Build history of the part. All positions in model axes, mm. Give positions to 0.01 mm unless a question says otherwise; leave off trailing zeros. Order: outer loops, then holes, each group sorted by start corner. A loop starts at its lowest first (then second) coordinate and runs counter-clockwise, first axis right, second up. Notation, with made-up numbers: M -5,28 L 44,28 A12 ccw 44,46 Z; hole C -38.5,84.25 d2. An arc over 180 degrees is marked long. Use CSV: the item, a comma, the result in double quotes. Start each with the question number.
Item 1: Wall check: line 1 along Y through (x, z) = (-2, -2.75); line 2 along X through (y, z) = (3.4, 2.5); line 3 along Z through (x, y) = (6.25, 0.2). Give the ranges that are in metal, low to high.
Item 2: Band-saw the part on A-A on z = 3. Write the cut outline in (x, y), plus the area to 3 significant figures.
Item 3: Pin check, flat tips, straight feed: P1, Ø2, axis at y = 3.5, z = 4, coming from the -X side; P2, Ø1, axis at x = 3.5, y = 1.5, coming from the -Z side; P3, Ø1.5, axis at x = 1.5, z = 4, coming from the -Y side; P4, Ø1.5, axis at y = 1, z = -4, coming from the -X side. Stop position of each tip, or through.
Item 4: Band-saw the part on D-D on y = 1.35. Write the cut outline in (x, z), plus the area to 3 significant figures.
Item 5: Two-plate mould, pull along X, no slides. Class faces 1 (the flat face through (0, 0.356, 0)), 2 (the cylindrical face through (0, 0.2, 2.7)), 3 (the flat face through (9.017, 3, 0)): pulls with the +X half, pulls with the -X half, needs draft (parallel to the pull), parting line crosses it, or undercut.
Item 6: Band-saw the part on C-C on x = -7.5. Write the cut outline in (y, z), plus the area to 3 significant figures.
Item 7: Band-saw the part on B-B on z = 0. Write the cut outline in (x, y).
from build123d import *

# Parameters (mm, degrees)
SKETCH1_W           = 18.796
SKETCH1_H           = 9.906
BOSS_EXTRUDE1_DEPTH = 0.3556
SKETCH2_R           = 2.25425
SKETCH2_W           = 5.08
SKETCH2_H           = 1.397
CUT_EXTRUDE1_DEPTH  = 11.629255118
SKETCH3_W           = 0.381
SKETCH3_H           = 7.112
BOSS_EXTRUDE2_DEPTH = 4.4196
FILLET2_R           = 0.508


with BuildPart() as part:
    # Sketch1 → Boss-Extrude1 (new body)
    with BuildSketch(Plane(origin=(0, 0, 0), x_dir=(1, 0, 0), z_dir=(0, 1, 0))):
        Rectangle(SKETCH1_W, SKETCH1_H)
    extrude(amount=BOSS_EXTRUDE1_DEPTH)

    # Sketch2 → Cut-Extrude1 (cut, through all)
    with BuildSketch(Plane(origin=(0, 0.3556, 0), x_dir=(1, 0, 0), z_dir=(0, 1, 0))):
        with Locations((0, 4.953)):
            Circle(SKETCH2_R)
        with Locations((0, -4.953)):
            Circle(SKETCH2_R)
        with Locations((-6.858, 4.2545)):
            Rectangle(SKETCH2_W, SKETCH2_H)
        with Locations((6.858, -4.2545)):
            Rectangle(SKETCH2_W, SKETCH2_H)
        with Locations((6.858, 4.2545)):
            Rectangle(SKETCH2_W, SKETCH2_H)
        with Locations((-6.858, -4.2545)):
            Rectangle(SKETCH2_W, SKETCH2_H)
    extrude(amount=-CUT_EXTRUDE1_DEPTH, mode=Mode.SUBTRACT)

    # Sketch3 → Boss-Extrude2 (add)
    with BuildSketch(Plane(origin=(0, 0.3556, 0), x_dir=(1, 0, 0), z_dir=(0, 1, 0))):
        with Locations((9.2075, 0)):
            Rectangle(SKETCH3_W, SKETCH3_H)
    extrude(amount=BOSS_EXTRUDE2_DEPTH)

    # Fillet2
    fillet2_edges = [part.edges().sort_by_distance(p)[0] for p in [
        (9.398, 0, 0),
    ]]
    fillet(fillet2_edges, radius=FILLET2_R)


solid = part.part
Model answer:
1,line 1,"y = 0 to 0.36"
1,line 2,"x = 9.02 to 9.4"
1,line 3,"z = -3.56 to 3.56"
2,outline,"M -9.4,0 L -1.13,0 L -1.13,0.36 L -9.4,0.36 Z; M 1.13,0 L 8.89,0 A0.51 ccw 9.4,0.51 L 9.4,4.78 L 9.02,4.78 L 9.02,0.36 L 1.13,0.36 Z"
2,area,"7.51 mm^2"
3,P1,"stops at x = 9.02"
3,P2,"passes through"
3,P3,"stops at y = 0"
3,P4,"stops at x = -4.32"
4,outline,"M 9.02,-3.56 L 9.4,-3.56 L 9.4,3.56 L 9.02,3.56 Z"
4,area,"2.71 mm^2"
5,face 1,"needs draft"
5,face 2,"undercut"
5,face 3,"pulls with the -X half"
6,outline,"M 0,-3.56 L 0.36,-3.56 L 0.36,3.56 L 0,3.56 Z"
6,area,"2.53 mm^2"
7,outline,"M -9.4,0 L 8.89,0 A0.51 ccw 9.4,0.51 L 9.4,4.78 L 9.02,4.78 L 9.02,0.36 L -9.4,0.36 Z"
